Source: CAD feature listing. Evaluate the final solid. Frame: model axes, mm. Give positions to 0.01 mm unless a question says otherwise; leave off trailing zeros. Write each loop counter-clockwise with the first axis right and the second up, starting at its lowest first coordinate (ties: lowest second). Pieces come first, ordered by that corner, then holes. Notation, with made-up numbers: M 48.5,-25 L 60.5,-25 A21 cw 60.5,-19 Z; hole C -30,4 d6. An arc over 180 degrees is marked long. Return JSON: item names as keys, results as strings.
```python
from build123d import *


with BuildPart() as f1:
    # F0 (on Front) → F1 (revolve)
    with BuildSketch(Plane.XZ):
        with BuildLine():
            Line((-29.032616, -77.086337), (0, -77.086337))
            Line((0, -77.086337), (0, 79.64943))
            Line((0, 79.64943), (-12.292725, 79.64943))
            ThreePointArc((-12.292725, 79.64943), (-39.233493, 68.490199), (-50.392725, 41.54943))
            Line((-50.392725, 41.54943), (-50.392725, -6.453492))
            Line((-50.392725, -6.453492), (-6.416031, -6.453492))
            Line((-6.416031, -6.453492), (-6.416031, -68.201698))
            Line((-6.416031, -68.201698), (-29.032616, -68.201698))
            Line((-29.032616, -68.201698), (-29.032616, -77.086337))
        make_face()
    revolve(axis=Axis((0, 0, 1.281547), (0, 0, -1)))


solid = f1.part
```
1) Line query: line 1 (Y direction, x = 0, z = 18); line 2 (X direction, y = -1.5, z = 27.5); line 3 (Z direction, x = -12, y = 0). Output: solid intervals per line, ascending. Write a range as [from, to].
Numbers:
{"line 1": "y = [-50.39, 50.39]", "line 2": "x = [-50.37, 50.37]", "line 3": "z = [-77.09, -68.2], [-6.45, 79.65]"}
2) Cut plane B-B, the plane z = -58. Return the cut outline in (x, y), then the cut area to 3 significant figures.
Numbers:
{"outline": "C 0,0 d12.83", "area": "129 mm²"}
3) Cut plane A-A, the plane z = 9.5. Return the cut outline in (x, y), then the cut area to 3 significant figures.
Numbers:
{"outline": "C 0,0 d100.79", "area": "7,980 mm²"}
4) Draft query along Z for faces 1 (the face through (6.294, -28.342, -72.706)), 2 (the face through (4.729, 4.336, -37.76)), 3 (the face through (0, 0, 79.649)). Return one class per face: released by +Z, released by -Z, zero draft, split by the parting line, or undercut.
Numbers:
{"face 1": "zero draft", "face 2": "undercut", "face 3": "released by +Z"}
5) Contact query for flat-ended pins moving along their axis: pin 1 Ø10 at (y, z) = (22.5, -10) entering from -X; pin 2 Ø4 at (x, z) = (6, 60) entering from -Y; pin 3 Ø5 at (y, z) = (26.5, 27.5) entering from +X. Output: stop coordinate, or through.
Numbers:
{"pin 1": "stops at x = -46.68", "pin 2": "stops at y = -46.3", "pin 3": "stops at x = 44.31"}
